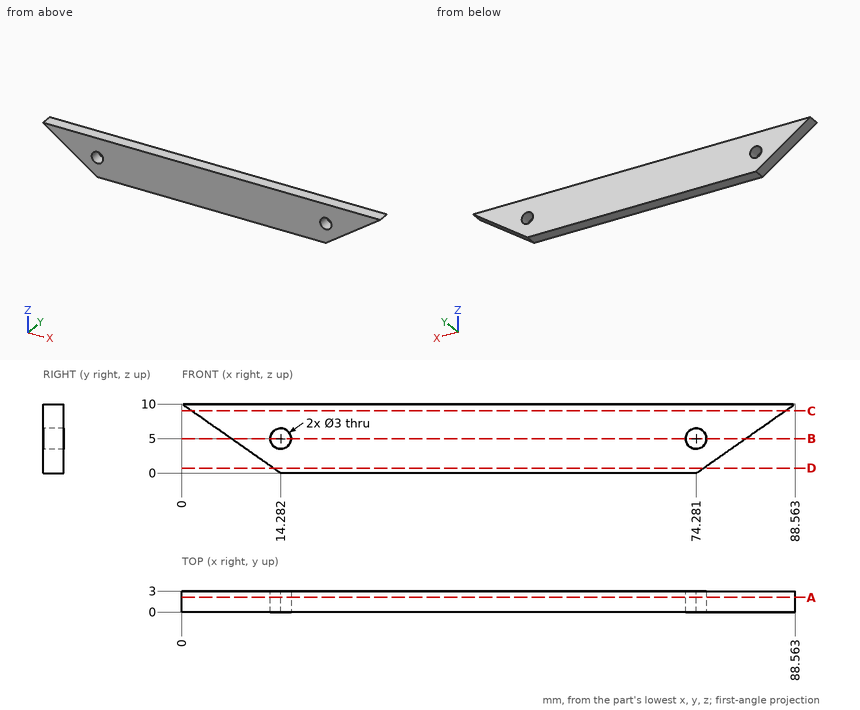
Design review of the part shown in the three views and the two pictorial views. Dimensions are in mm from the part's minimum x, y and z. Round coordinates to 2 decimals unless told otherwise and drop trailing zeros. Write each loop counter-clockwise with the first axis right and the second up, starting at its lowest first coordinate (ties: lowest second). Pieces come first, ordered by that corner, then holes. Notation, with made-up numbers: (-17.75, -33) - (27.25, -33) arc R22 cw to (27.25, -1) - close; hole circle Ø7 at (-26, 57). An arc over 180 degrees is marked (long way). Return JSON: item names as keys, results as strings. Group by question number.
Item 1: We need section A-A on y = 2.1. Write out the cut boundary in (x, z).
Item 2: For probe 1 along X at (y, z) = (2.45, 5) (1 decimal); probe 2 along Z at (x, y) = (73.5, 2.6); probe 3 along Z at (x, y) = (5, 2.35), list the stretches that pass through material, from the lowest coordinate up. Write a range as [from, to].
Item 3: We need section D-D on z = 0.75. Write out the cut boundary in (x, y).
Item 4: We need section B-B on z = 5. Write out the cut boundary in (x, y), and give its area (3 significant figures).
Item 5: We need section C-C on z = 9. Write out the cut boundary in (x, y) (1 decimal).
Model answer:
{
 "1": {"outline": "(0, 10) - (14.28, 0) - (74.28, 0) - (88.56, 10) - close; hole circle Ø3 at (14.28, 5); hole circle Ø3 at (74.28, 5)"},
 "2": {"probe 1": "x = [7.1, 12.8], [15.8, 72.8], [75.8, 81.4]", "probe 2": "z = [0, 3.72], [6.28, 10]", "probe 3": "z = [6.5, 10]"},
 "3": {"outline": "(13.21, 0) - (75.35, 0) - (75.35, 3) - (13.21, 3) - close"},
 "4": {"outline": "(7.14, 0) - (12.78, 0) - (12.78, 3) - (7.14, 3) - close; (15.78, 0) - (72.78, 0) - (72.78, 3) - (15.78, 3) - close; (75.78, 0) - (81.42, 0) - (81.42, 3) - (75.78, 3) - close", "area": "205 mm²"},
 "5": {"outline": "(1.4, 0) - (87.1, 0) - (87.1, 3) - (1.4, 3) - close"}
}
